Print and shaded views of the part. All mm, measured from the part's lowest x, y and z. A direction names the side the tool comes from. Round coordinates to 2 decimals unless told otherwise and drop trailing zeros. Loops run counter-clockwise (first coordinate to the right, second up) from the corner with the lowest first, then second, coordinate; pieces in that order, holes last. Notation, with made-up numbers: (79, 40) - (108, 40) arc R17 ccw to (108, 50) - close; hole circle Ø2 at (69.5, 34). An arc over 180 degrees is marked (long way). Use one line per item in the form item = value.
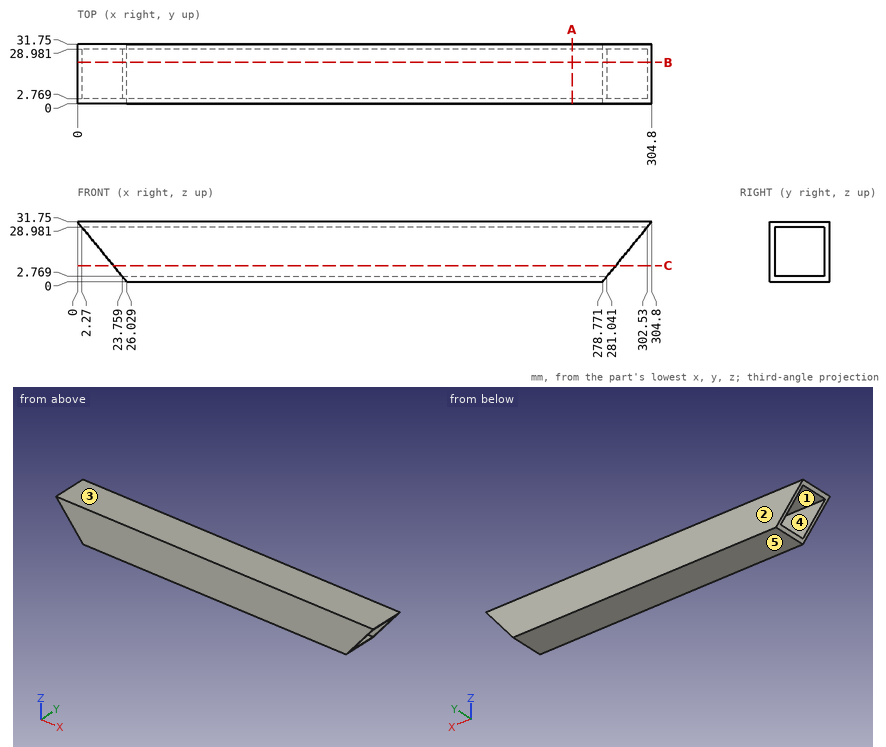
1. Tool access for the marked faces 1 and 2: list every direction of +Z, -Z, +X, -X, +Y, -Y with a clear straight run to the whole face (end or side of a thin tool).
Geometry check:
face_1 = +X, -X
face_2 = +Z, -Z, +X, -X, +Y
2. Cut at B-B, the plane y = 22. Give the cut face in (x, z).
Geometry check:
outline = (0, 31.75) - (2.27, 28.98) - (302.53, 28.98) - (304.8, 31.75) - close; (23.76, 2.77) - (26.03, 0) - (278.77, 0) - (281.04, 2.77) - close
3. Pull direction Z, two halves, no side cores. Call the marked faces 3, 4 and 5: +Z half, -Z half, draft (parallel to the pull), parting line (faces both ways), or undercut.
Geometry check:
face_3 = +Z half
face_4 = undercut
face_5 = -Z half
4. Wall check: probe 1 along Z at (x, y) = (53, 7); probe 2 along Z at (x, y) = (290, 5.5). Give the ranges that are in metal, low to high.
Geometry check:
probe_1 = 0 to 2.77, 28.98 to 31.75
probe_2 = 28.98 to 31.75
5. Flat gauge pin, fed straight in: pin 1 (8 mm diameter, centred on x = 237, y = 15.5, fed in from -Z). Where does the tip first touch, or does it go through?
Geometry check:
pin_1 = 0
6. Cut at C-C, the plane z = 8.5. Give the cut face in (x, y), plus the area to 3 significant figures.
Geometry check:
outline = (19.06, 0) - (285.74, 0) - (285.74, 2.77) - (19.06, 2.77) - close; (19.06, 28.98) - (285.74, 28.98) - (285.74, 31.75) - (19.06, 31.75) - close
area = 1,480 mm^2
7. Cut at A-A, the plane x = 262.5. Give the cut face in (y, z), plus the area to 3 significant figures.
Geometry check:
outline = (0, 0) - (31.75, 0) - (31.75, 31.75) - (0, 31.75) - close; hole (2.77, 2.77) - (28.98, 2.77) - (28.98, 28.98) - (2.77, 28.98) - close
area = 321 mm^2
